Here's how the part is built. I have some questions about the finished solid (model axes, mm). Face numbers are marked on the shaded views. A direction names the side the tool comes from. Give positions to 0.01 mm unless a question says otherwise; leave off trailing zeros. Loops run counter-clockwise (first coordinate to the right, second up) from the corner with the lowest first, then second, coordinate; pieces in that order, holes last.
Q1. Suppose I cut it at D-D (z = -26). List the corners of the cut face in (x, y) for me.
Q2. Thinking about a two-plate mould opening in X: for the marked faces 1, 2, 3 and 4, which applies, pulls with the +X half, pulls with the -X half, needs draft (parallel to the pull), parting line crosses it, or undercut?
Q3. Suppose I cut it at C-C (y = 1.25). List the corners of the cut face in (x, z) for me.
Q4. For the marked faces 5, 6, 7 and 8, which set-ups out of +Z, -Z, +X, -X, +Y, -Y let a thin tool reach every point of the face, with its end or its side?
Q5. I'm going to push flat-ended pins straight in: P1, Ø1, axis at x = -2.5, z = -23.5, coming from the -Y side; P2, Ø4, axis at x = -1.5, z = 5, coming from the +Y side; P3, Ø6.5, axis at x = 2, z = 3, coming from the -Y side; P4, Ø5, axis at x = 2, y = 0, coming from the +Z side. Where does each tip first touch, or does it pass through?
Q6. Suppose I cut it at A-A (z = 2.5). List the corners of the cut face in (x, y) for me, and give its area (3 significant figures).
Q7. Suppose I cut it at B-B (x = -2). List the corners of the cut face in (y, z) for me, and give its area (3 significant figures).
Q8. I need wall thicknesses on probe 1 along Y at (x, z) = (-3, 6); probe 2 along X at (y, z) = (2.5, -19); probe 3 along Z at (x, y) = (-5, -2.75). Which ranges of each line are inside material? Lowest first, please.
```python
from build123d import *

# Parameters (mm, degrees)
SKETCH1_W           = 12.04
SKETCH1_H           = 7.58
SKETCH1_W_2         = 8.04
SKETCH1_H_2         = 3.58
BOSS_EXTRUDE1_DEPTH = 8
SKETCH1_2_W         = 12.04
SKETCH1_2_H         = 7.58
SKETCH1_2_W_2       = 8.04
SKETCH1_2_H_2       = 3.58
BOSS_EXTRUDE2_DEPTH = 2
EXTRUDE_THIN1_START = -12.04
EXTRUDE_THIN1_DEPTH = 12.04
SKETCH5_W           = 12.04
SKETCH5_H           = 7.58
SKETCH5_W_2         = 8.04
SKETCH5_H_2         = 3.58
BOSS_EXTRUDE4_DEPTH = 10
SKETCH5_4_W         = 12.04
SKETCH5_4_H         = 7.58
BOSS_EXTRUDE5_DEPTH = 2
CHAMFER1_SIZE       = 1.5


with BuildPart() as part:
    # Sketch1 → Boss-Extrude1 (new body)
    with BuildSketch(Plane.XY):
        Rectangle(SKETCH1_W, SKETCH1_H)
        Rectangle(SKETCH1_W_2, SKETCH1_H_2, mode=Mode.SUBTRACT)
    extrude(amount=BOSS_EXTRUDE1_DEPTH)

    # Sketch1<2> → Boss-Extrude2 (add)
    # profile 1 of 2: a face of its own
    with BuildSketch(Plane.XY):
        Rectangle(SKETCH1_2_W, SKETCH1_2_H)
        Rectangle(SKETCH1_2_W_2, SKETCH1_2_H_2, mode=Mode.SUBTRACT)
    # profile 2 of 2: a face of its own
    with BuildSketch(Plane.XY):
        Rectangle(SKETCH1_2_W_2, SKETCH1_2_H_2)
    extrude(amount=-BOSS_EXTRUDE2_DEPTH)

    # Sketch3 → Extrude-Thin1 (add)
    with BuildSketch(Plane(origin=(6.02, 9.81, 0), x_dir=(0, -1, 0), z_dir=(1, 0, 0)).offset(EXTRUDE_THIN1_START)):
        with BuildLine():
            Line((13.6, 2), (15.597169895, 2))
            ThreePointArc((15.597169895, 2), (16.306275023, 2.294897229), (16.597153876, 3.005660165))
            ThreePointArc((16.597153876, 3.005660165), (16.430894398, 9.75), (16.008713261, 16.483166054))
            ThreePointArc((16.008713261, 16.483166054), (15.656994218, 17.16587256), (14.924885462, 17.397845032))
            Line((14.924885462, 17.397845032), (12.935315402, 17.223780206))
            Line((12.935315402, 17.223780206), (12.761003916, 19.216169602))
            Line((12.761003916, 19.216169602), (14.750573976, 19.390234428))
            ThreePointArc((14.750573976, 19.390234428), (16.946900244, 18.694317012), (18.002057373, 16.646197494))
            ThreePointArc((18.002057373, 16.646197494), (18.428990842, 9.837238775), (18.597121838, 3.016980496))
            ThreePointArc((18.597121838, 3.016980496), (17.724485279, 0.884691688), (15.597169895, 0))
            Line((15.597169895, 0), (13.6, 0))
            Line((13.6, 0), (13.6, 2))
        make_face()
    extrude(amount=EXTRUDE_THIN1_DEPTH)



with BuildPart() as body_2:
    # Sketch5 → Boss-Extrude4 (new body)
    with BuildSketch(Plane(origin=(0, -2.104915883, -19.142146491), x_dir=(1, 0, 0), z_dir=(0, -0.08715574274765182, 0.9961946980917462))):
        with Locations((0, 2.940680048)):
            Rectangle(SKETCH5_W, SKETCH5_H)
        with Locations((0, 2.940680048)):
            Rectangle(SKETCH5_W_2, SKETCH5_H_2, mode=Mode.SUBTRACT)
    extrude(amount=-BOSS_EXTRUDE4_DEPTH)


with BuildPart() as part_1:
    add(part.part)

    add(body_2.part)  # Boss-Extrude5 merges body 2
    # Sketch5<4> → Boss-Extrude5 (add)
    with BuildSketch(Plane(origin=(0, -2.104915883, -19.142146491), x_dir=(1, 0, 0), z_dir=(0, -0.08715574274765182, 0.9961946980917462))):
        with Locations((0, 2.940680048)):
            Rectangle(SKETCH5_4_W, SKETCH5_4_H)
    extrude(amount=BOSS_EXTRUDE5_DEPTH)

    # Chamfer1
    chamfer1_edges = [part_1.edges().sort_by_distance(p)[0] for p in [
        (6.02, -2.515225202, -24.197143093),
        (-6.02, -2.515225202, -24.197143093),
        (0, 3.79, -2),
        (6.02, -3.79, 4),
        (-6.02, -3.79, 4),
        (-6.02, 3.79, 3),
        (6.02, 3.79, 3),
        (0, 4.42584041, -16.563139676),
        (6.02, 4.948774866, -22.540307865),
        (-6.02, 4.948774866, -22.540307865),
    ]]
    chamfer(chamfer1_edges, length=CHAMFER1_SIZE)


solid = part_1.part
```
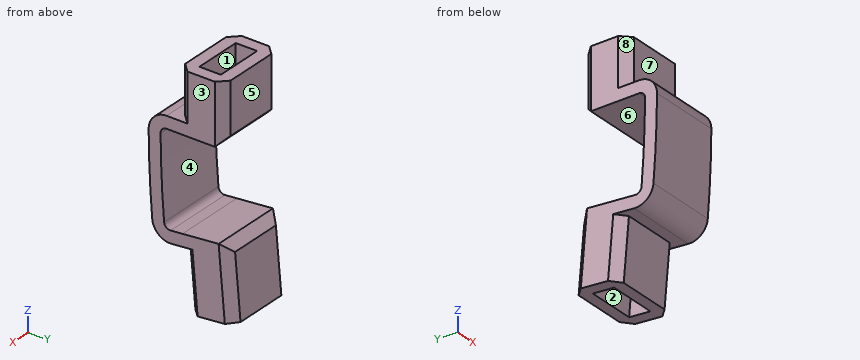
Solutions:
1. outline: (-6.02, -0.85) - (-4.52, -2.36) - (4.52, -2.36) - (6.02, -0.85) - (6.02, 3.75) - (4.52, 5.25) - (-4.52, 5.25) - (-6.02, 3.75) - close; hole (-4.02, -0.35) - (4.02, -0.35) - (4.02, 3.24) - (-4.02, 3.24) - close
2. face 1: undercut
2. face 2: undercut
2. face 3: pulls with the +X half
2. face 4: needs draft
3. outline: (-6.02, -28.89) - (-4.02, -28.89) - (-4.02, -18.85) - (4.02, -18.85) - (4.02, -28.89) - (6.02, -28.89) - (6.02, -16.84) - (-6.02, -16.84) - close; (-6.02, -2) - (6.02, -2) - (6.02, 8) - (4.02, 8) - (4.02, 0) - (-4.02, 0) - (-4.02, 8) - (-6.02, 8) - close
4. face 5: +Z, +X, -X, +Y
4. face 6: +X, -X, +Y
4. face 7: +Z, +X, -X, -Y
4. face 8: +Z, -X, -Y
5. P1: stops at y = -2.62
5. P2: stops at y = 3.79
5. P3: stops at y = -6.99
5. P4: stops at z = 8
6. outline: (-6.02, -2.29) - (-4.52, -3.79) - (4.52, -3.79) - (6.02, -2.29) - (6.02, 2.29) - (4.52, 3.79) - (-4.52, 3.79) - (-6.02, 2.29) - close; hole (-4.02, -1.79) - (4.02, -1.79) - (4.02, 1.79) - (-4.02, 1.79) - close
6. area: 58.0 mm2
7. outline: (-8.79, -3.02) arc R179.67 ccw to (-8.19, -16.65) arc R3 ccw to (-4.94, -19.39) - (-2.95, -19.22) - (-2.08, -29.18) - (-0.09, -29) - (-0.96, -19.04) - (2.61, -18.73) - (3.48, -28.69) - (5.47, -28.52) - (4.56, -18.06) - (2.93, -16.69) - (-5.11, -17.4) arc R1 cw to (-6.2, -16.48) arc R177.67 cw to (-6.79, -3.01) arc R1 cw to (-5.79, -2) - (2.29, -2) - (3.79, -0.5) - (3.79, 8) - (1.79, 8) - (1.79, 0) - (-1.79, 0) - (-1.79, 8) - (-3.79, 8) - (-3.79, 0) - (-5.79, 0) arc R3 ccw to start
7. area: 148 mm2
8. probe 1: y = -3.79 to -1.79, 1.79 to 3.79
8. probe 2: x = -6.02 to -4.02, 4.02 to 6.02
8. probe 3: z = -19.2 to -17.19, -2 to 8
